Could you check a few things on this model? Use its own coordinates, in mm. A direction names the side the tool comes from. Round coordinates to 2 decimals unless told otherwise and drop trailing zeros. Order: outer loops, then holes, each group sorted by start corner. A loop starts at its lowest first (then second) coordinate and runs counter-clockwise, first axis right, second up. Notation, with made-up numbers: (59.5, 65.5) - (110.5, 65.5) arc R18 ccw to (110.5, 87.5) - close; hole circle Ø10 at (87, 25.25). An arc over 180 degrees is marked (long way). Return JSON: item names as keys, results as strings. Group by question number.
from build123d import *

# Parameters (mm, degrees)
SKETCH1_R             = 5
BOSS_EXTRUDE1_DEPTH   = 25
SKETCH2_W             = 5
SKETCH2_H             = 15
BOSS_EXTRUDE2_DEPTH   = 5
SKETCH3_W             = 5
SKETCH3_H             = 15
BOSS_EXTRUDE3_DEPTH   = 2.5
SKETCH5_W             = 5
SKETCH5_H             = 15
BOSS_EXTRUDE5_DEPTH   = 2.5
BOSS_EXTRUDE6_START   = 25
SKETCH6_R             = 5
BOSS_EXTRUDE6_DEPTH   = 25
SKETCH7_W             = 5
SKETCH7_H             = 15
BOSS_EXTRUDE7_DEPTH   = 5
F_5_0MM_DOWEL_HOLE1_D = 5
BOSS_EXTRUDE8_START   = 20
SKETCH14_R            = 5
BOSS_EXTRUDE8_DEPTH   = 20
SKETCH15_R            = 5
BOSS_EXTRUDE9_DEPTH   = 50.04395072
SKETCH18_W            = 5
SKETCH18_H            = 15
BOSS_EXTRUDE10_DEPTH  = 5


with BuildPart() as part:
    # Sketch1 → Boss-Extrude1 (new body)
    with BuildSketch(Plane.XY):
        with Locations(Location((0, 0, 0), (0, 0, 180))):
            Circle(SKETCH1_R)
    extrude(amount=BOSS_EXTRUDE1_DEPTH)

    # Sketch2 → Boss-Extrude2 (add)
    with BuildSketch(Plane.XY.offset(25)):
        Rectangle(SKETCH2_W, SKETCH2_H)
    extrude(amount=-BOSS_EXTRUDE2_DEPTH)

    # Sketch3 → Boss-Extrude3 (add)
    with BuildSketch(Plane(origin=(0, 0, 0), x_dir=(-1, 0, 0), z_dir=(0, 0, -1))):
        Rectangle(SKETCH3_W, SKETCH3_H)
    extrude(amount=-BOSS_EXTRUDE3_DEPTH)

    # Sketch5 → Boss-Extrude5 (add)
    with BuildSketch(Plane(origin=(0, 0, 0), x_dir=(-1, 0, 0), z_dir=(0, 0, -1))):
        Rectangle(SKETCH5_W, SKETCH5_H)
    extrude(amount=BOSS_EXTRUDE5_DEPTH)

    # Sketch6 → Boss-Extrude6 (add)
    with BuildSketch(Plane(origin=(0, 0, 0), x_dir=(-1, 0, 0), z_dir=(0, 0, -1)).offset(BOSS_EXTRUDE6_START)):
        Circle(SKETCH6_R)
    extrude(amount=-BOSS_EXTRUDE6_DEPTH)

    # Sketch7 → Boss-Extrude7 (add)
    with BuildSketch(Plane(origin=(0, 0, -25), x_dir=(-1, 0, 0), z_dir=(0, 0, -1))):
        Rectangle(SKETCH7_W, SKETCH7_H)
    extrude(amount=-BOSS_EXTRUDE7_DEPTH)

    # Ø5.0mm Dowel Hole1 (through all)
    with Locations(Plane.XY.offset(25)):
        with Locations((0, 0)):
            Hole(F_5_0MM_DOWEL_HOLE1_D / 2)

    # Sketch14 → Boss-Extrude8 (add)
    with BuildSketch(Plane(origin=(0, 0, -25), x_dir=(-1, 0, 0), z_dir=(0, 0, -1)).offset(BOSS_EXTRUDE8_START)):
        Circle(SKETCH14_R)
    extrude(amount=-BOSS_EXTRUDE8_DEPTH)

    # Sketch15 → Boss-Extrude9 (add)
    with BuildSketch(Plane.XY.offset(25)):
        with Locations(Location((0, 0, 0), (0, 0, 180))):
            Circle(SKETCH15_R)
    extrude(amount=BOSS_EXTRUDE9_DEPTH)

    # Sketch18 → Boss-Extrude10 (add)
    with BuildSketch(Plane.XY.offset(75.04395072)):
        Rectangle(SKETCH18_W, SKETCH18_H)
    extrude(amount=-BOSS_EXTRUDE10_DEPTH)


solid = part.part
1) For faces 5 (the flat face through (2.5, 6, 0)), 6 (the flat face through (-2.5, 6, 0)), 7 (the flat face through (2.5, -6, -23)), 8 (the flat face through (0, 0, -25)), 9 (the flat face through (-2.5, -6, 73)), which set-ups out of +Z, -Z, +X, -X, +Y, -Y let a thin tool reach every point of the face, with its end or its side?
2) I want a section at A-A, the plane y = -6. List the corners of the cut face in (x, z) for me.
3) We'd pull the mould along Y, two halves only. Please class faces 1 (the cylindrical face through (0.54, -2.44, -0.35)), 2 (the flat face through (-2.5, 6, -23)), 3 (the flat face through (0, 7.5, -23)), 4 (the flat face through (0, -7.5, 23)): +Y half, -Y half, draft (parallel to the pull), parting line (faces both ways), or undercut.
4) If I drill on line 1 along Z through (x, y) = (-1.5, 6.75); line 2 along Y through (x, z) = (0, -13.5); line 3 along Z through (x, y) = (-0.5, -2.25), over which ranges is the centre line in solid material (lowest first)? Write a range as from..to.
5) Will these pins go through, and if not, where does the flat tip stop? pin 1 (3.5 mm diameter, centred on y = 6, z = 72.5, fed in from -X); pin 2 (1.5 mm diameter, centred on y = 4.5, z = -31.5, fed in from -X); pin 3 (1 mm diameter, centred on y = 6, z = -23.5, fed in from +X).
6) I want a section at C-C, the plane z = 17. List the corners of the cut face in (x, y) for me.
7) I want a section at D-D, the plane z = 53. List the corners of the cut face in (x, y) for me.
8) I want a section at B-B, the plane y = 0. List the corners of the cut face in (x, z) for me, plus the area to 3 significant figures.
Outcome:
{
 "1": {"face 5": "+Z, -Z, +X, +Y", "face 6": "+Z, -Z, -X, +Y", "face 7": "+Z, -Z, +X, -Y", "face 8": "none", "face 9": "+Z, -Z, -X, -Y"},
 "2": {"outline": "(-2.5, -25) - (2.5, -25) - (2.5, -20) - (-2.5, -20) - close; (-2.5, -2.5) - (2.5, -2.5) - (2.5, 2.5) - (-2.5, 2.5) - close; (-2.5, 20) - (2.5, 20) - (2.5, 25) - (-2.5, 25) - close; (-2.5, 70.04) - (2.5, 70.04) - (2.5, 75.04) - (-2.5, 75.04) - close"},
 "3": {"face 1": "undercut", "face 2": "draft", "face 3": "+Y half", "face 4": "-Y half"},
 "4": {"line 1": "-25..-20, -2.5..2.5, 20..25, 70.04..75.04", "line 2": "-5..-2.5, 2.5..5", "line 3": "-45..-25, 25..75.04"},
 "5": {"pin 1": "x = -2.63", "pin 2": "x = -3.31", "pin 3": "x = 2.5"},
 "6": {"outline": "circle Ø10 at (0, 0); hole circle Ø5 at (0, 0)"},
 "7": {"outline": "circle Ø10 at (0, 0)"},
 "8": {"outline": "(-5, -45) - (5, -45) - (5, 75.04) - (-5, 75.04) - close; hole (-2.5, -25) - (2.5, -25) - (2.5, 25) - (-2.5, 25) - close", "area": "950 mm^2"}
}
